```python
from build123d import *

# Parameters (mm, degrees)
F0_W     = 46.089629
F0_H     = 79.049881
F1_DEPTH = 25.4
F2_R     = 17.749963
F3_DEPTH = 25.4
F4_R     = 11.375328
F5_DEPTH = 50.801


with BuildPart() as f1:
    # F0 (on Right) → F1 (new body)
    with BuildSketch(Plane.YZ):
        with Locations((3.503773, -7.040882)):
            Rectangle(F0_W, F0_H)
    extrude(amount=F1_DEPTH)

    # F2 (on face) → F3 (join)
    with BuildSketch(Plane(origin=(0, 0, 0), x_dir=(0, -1, 0), z_dir=(-1, 0, 0))):
        with Locations((-5.44068, -3.68046)):
            Circle(F2_R)
    extrude(amount=F3_DEPTH)

    # F4 (on face) → F5 (cut, through all)
    with BuildSketch(Plane(origin=(-25.4, 0, 0), x_dir=(0, -1, 0), z_dir=(-1, 0, 0))):
        with Locations((-5.44068, -3.68046)):
            Circle(F4_R)
    extrude(amount=-F5_DEPTH, mode=Mode.SUBTRACT)


solid = f1.part
```
CAD build for the part. Positions are in the model's coordinates, mm. A direction names the side the tool comes from. Round coordinates to 2 decimals unless told otherwise and drop trailing zeros. Order: outer loops, then holes, each group sorted by start corner. A loop starts at its lowest first (then second) coordinate and runs counter-clockwise, first axis right, second up. Notation, with made-up numbers: (44.5, 19.25) - (82.5, 19.25) arc R21 ccw to (82.5, 47.25) - close; hole circle Ø8 at (-3, 79.5). An arc over 180 degrees is marked (long way). Answer as CSV lines item,"result". Start each with the question number.
1. Saw through at A-A, the plane y = -4.5. Write the cut outline in (x, z).
2. Saw through at B-B, the plane z = -10. Write the cut outline in (x, y).
3. Saw through at D-D, the plane x = 12. Write the cut outline in (y, z).
4. Pin check, flat tips, straight feed: pin 1 (10 mm diameter, centred on y = 15, z = -9.5, fed in from +X); pin 2 (3 mm diameter, centred on x = -17.5, z = 6.5, fed in from -Y). Stop position of each tip, or through.
5. Drill centre lines: L1, parallel to Z at x = -12.5, y = 5.5; L2, parallel to X at y = -17, z = 7.5; L3, parallel to Z at x = -9, y = 14.5. Where is each one in solid material? Low to high. Write a range as [from, to].
6. Saw through at C-C, the plane z = -34.5. Write the cut outline in (x, y), and give its area (3 significant figures).
7. Pull direction Y, two halves, no side cores. Call faces 3 (the face through (13, 26.549, -8)), 4 (the face through (25.4, 3, -15)), 5 (the face through (-0.356, -5.067, -8.037)): +Y half, -Y half, draft (parallel to the pull), parting line (faces both ways), or undercut.
8. Tool access for faces 1 (the face through (13, 3, 32.484)), 2 (the face through (-12.52, -11.49, 1.65)): list every direction of +Z, -Z, +X, -X, +Y, -Y with a clear straight run to the whole face (end or side of a thin tool).
Model answer:
1,outline,"(-25.4, -18.39) - (0, -18.39) - (0, -46.57) - (25.4, -46.57) - (25.4, -9.21) - (-25.4, -9.21) - close; (-25.4, 1.85) - (25.4, 1.85) - (25.4, 32.48) - (0, 32.48) - (0, 11.02) - (-25.4, 11.02) - close"
2,outline,"(-25.4, -11.15) - (0, -11.15) - (0, -19.54) - (25.4, -19.54) - (25.4, -4.02) - (-25.4, -4.02) - close; (-25.4, 14.9) - (25.4, 14.9) - (25.4, 26.55) - (0, 26.55) - (0, 22.03) - (-25.4, 22.03) - close"
3,outline,"(-19.54, -46.57) - (26.55, -46.57) - (26.55, 32.48) - (-19.54, 32.48) - close; hole circle Ø22.75 at (5.44, -3.68)"
4,pin 1,"stops at x = 25.4"
4,pin 2,"stops at y = -10.04"
5,L1,"z = [-21.43, -15.06], [7.69, 14.07]"
5,L2,"x = [0, 25.4]"
5,L3,"z = [-18.94, -10.56], [3.2, 11.58]"
6,outline,"(0, -19.54) - (25.4, -19.54) - (25.4, 26.55) - (0, 26.55) - close"
6,area,"1,170 mm²"
7,face 3,"+Y half"
7,face 4,"draft"
7,face 5,"undercut"
8,face 1,"+Z, +X, -X, +Y, -Y"
8,face 2,"-X"
